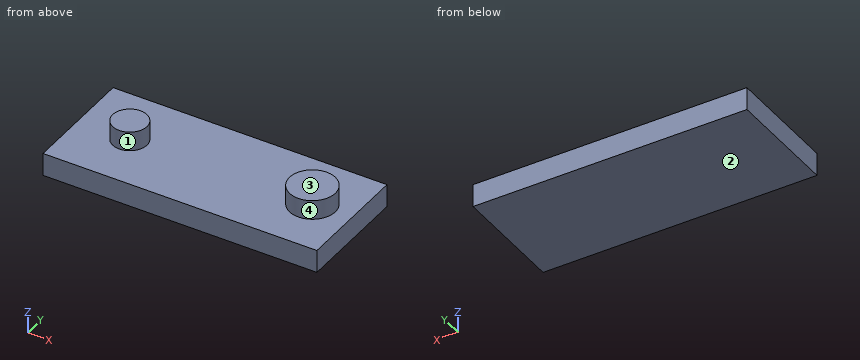
from build123d import *

# Parameters (mm, degrees)
SKETCH_1_W      = 120
SKETCH_1_H      = 50
EXTRUDE_1_DEPTH = 5
SKETCH_2_R      = 7.5
SKETCH_2_R_2    = 10
EXTRUDE_2_DEPTH = 8.5


with BuildPart() as part:
    # 草图1 → 凸台-拉伸1 (new, symmetric)
    with BuildSketch(Plane.XY):
        with Locations((34.086506066, 14.145511968)):
            Rectangle(SKETCH_1_W, SKETCH_1_H)
    extrude(amount=EXTRUDE_1_DEPTH, both=True)

    # 草图2 → 凸台-拉伸2 (add, symmetric)
    with BuildSketch(Plane.XY.offset(5)):
        with Locations((-3.130706557, 13.98825614)):
            Circle(SKETCH_2_R)
        with Locations((76.869293443, 13.98825614)):
            Circle(SKETCH_2_R_2)
    extrude(amount=EXTRUDE_2_DEPTH, both=True)


solid = part.part
Check sheet for the modelled part. Datum: model origin and axes. Units: mm. Face numbers are marked on the shaded views. A direction names the side the tool comes from. Round coordinates to 2 decimals unless told otherwise and drop trailing zeros. Order: outer loops, then holes, each group sorted by start corner. A loop starts at its lowest first (then second) coordinate and runs counter-clockwise, first axis right, second up. Notation, with made-up numbers: M 3.5,54.25 L 52.5,54.25 A35 cw 52.5,93.25 Z; hole C 26.25,63.5 d1. An arc over 180 degrees is marked long. One line per item, written item: value. Start each with the question number.
1. Section check A-A on x = -5. Enter the section's corners in (y, z).
2. Release check for a two-part mould opening along X. For the marked faces 3 and 4 record: released by +X, released by -X, zero draft, split by the parting line, or undercut.
3. Section check C-C on x = 79.5. Enter the section's corners in (y, z).
4. Scan lines: line 1 along Z through (x, y) = (62, 24); line 2 along X through (y, z) = (19.5, 7.25); line 3 along X through (y, z) = (19, 7.5). Record each from-to range of solid material in increasing order.
5. Section check B-B on y = 19. Enter the section's corners in (x, z).
6. Access from +Z, -Z, +X, -X, +Y, -Y to the whole of each face (thin tool, end or side, straight path). Record for the marked faces 1 and 2.
7. Gauge pin test, flat ends, axial feed: P1, Ø1, axis at x = -12, y = 20, coming from the +Z side; P2, Ø3, axis at x = 70, z = 8, coming from the -Y side. Record the tip position at first contact, or that the pin passes through.
8. Section check D-D on y = 0. Enter the section's corners in (x, z), and give its area (3 significant figures).
Results found:
1. outline: M -10.85,-5 L 39.15,-5 L 39.15,5 L 21.25,5 L 21.25,13.5 L 6.72,13.5 L 6.72,5 L -10.85,5 Z
2. face 3: zero draft
2. face 4: undercut
3. outline: M -10.85,-5 L 39.15,-5 L 39.15,5 L 23.64,5 L 23.64,13.5 L 4.34,13.5 L 4.34,5 L -10.85,5 Z
4. line 1: -5 to 5
4. line 2: -8.22 to 1.96, 68.53 to 85.21
4. line 3: -8.71 to 2.45, 68.22 to 85.52
5. outline: M -25.91,-5 L 94.09,-5 L 94.09,5 L 85.52,5 L 85.52,13.5 L 68.22,13.5 L 68.22,5 L 2.45,5 L 2.45,13.5 L -8.71,13.5 L -8.71,5 L -25.91,5 Z
6. face 1: +Z
6. face 2: -Z, +X, -X, +Y, -Y
7. P1: z = 5
7. P2: y = 5.55
8. outline: M -25.91,-5 L 94.09,-5 L 94.09,5 L -25.91,5 Z
8. area: 1,200 mm^2
